The model under review builds one solid part; all positions refer to its coordinate system, in mm. A direction names the side the tool comes from. Round coordinates to 2 decimals unless told otherwise and drop trailing zeros. Write each loop counter-clockwise with the first axis right and the second up, starting at its lowest first coordinate (ties: lowest second). Pieces come first, ordered by that corner, then holes. Notation, with made-up numbers: (-8.75, 11.5) -> (13.25, 11.5) arc R13 cw to (13.25, 18.5) -> close; hole circle Ø5 at (65.25, 79.25). An arc over 180 degrees is marked (long way). Return JSON: item names as keys, results as strings. Group by question number.
1. Clearance check with flat-ended pins moving along their axes: P1, Ø1.3, axis at x = 1, z = 11, coming from the -Y side; P2, Ø1.1, axis at x = -4.5, y = -1.5, coming from the -Z side; P3, Ø2, axis at x = -3, z = 10, coming from the +Y side. State where each tip first meets the part, or that it passes through.
2. Tool access review of faces 5 (the flat face through (4, -1, 12)), 6 (the flat face through (4.5, -1, 11)), 7 (the flat face through (-5, 0, 12)): name each direction out of +Z, -Z, +X, -X, +Y, -Y from which nothing blocks a thin tool from reaching the whole face with its end or side.
3. Take a section at B-B, the plane z = 10.75. Write out the cut boundary in (x, y), then the cut area to 3 significant figures.
4. Mouldability with a two-part tool opening along X and no side actions: class faces 1 (the cylindrical face through (0, 1, 11)), 2 (the flat face through (4.5, -2, 12.2)), 3 (the flat face through (5, 0, 12)), 4 (the flat face through (-4, -1, 12)) as pulls with the +X half, pulls with the -X half, needs draft (parallel to the pull), parting line crosses it, or undercut.
5. For line 1 along X through (y, z) = (-1.8, 12.65); line 2 along Y through (x, z) = (-3, 13.5); line 3 along Z through (x, y) = (0.25, 0.8), list the stretches that pass through material, from the lowest coordinate up. Write a range as from..to.
6. Take a section at C-C, the plane z = 11.75. Write out the cut boundary in (x, y), then the cut area to 3 significant figures.
7. Take a section at A-A, the plane y = -1.45. Write out the cut boundary in (x, z), then the cut area to 3 significant figures.
8. Take a section at D-D, the plane x = 3. Write out the cut boundary in (y, z).
from build123d import *

# Parameters (mm, degrees)
BOSS_EXTRUDE1_DEPTH = 2
BOSS_EXTRUDE2_DEPTH = 2


with BuildPart() as part:
    # Sketch1 → Boss-Extrude1 (new body)
    with BuildSketch(Plane(origin=(0, 0, 0), x_dir=(1, 0, 0), z_dir=(0, 1, 0))):
        with BuildLine():
            Line((-5, -9.797958971), (-5, -13.076696831))
            ThreePointArc((-5, -13.076696831), (0, -14), (5, -13.076696831))
            Line((5, -13.076696831), (5, -9.797958971))
            ThreePointArc((5, -9.797958971), (0, -11), (-5, -9.797958971))
        make_face()
    extrude(amount=BOSS_EXTRUDE1_DEPTH)

    # Sketch3 → Boss-Extrude2 (add)
    with BuildSketch(Plane.XZ):
        with BuildLine():
            Line((5, 13.076696831), (5, 11))
            Line((5, 11), (4, 11))
            Line((4, 11), (4, 13.416407865))
            ThreePointArc((4, 13.416407865), (4.503204514, 13.255985407), (5, 13.076696831))
        make_face()
        with BuildLine():
            Line((-5, 11), (-5, 13.076696831))
            ThreePointArc((-5, 13.076696831), (-4.503204514, 13.255985407), (-4, 13.416407865))
            Line((-4, 13.416407865), (-4, 11))
            Line((-4, 11), (-5, 11))
        make_face()
    extrude(amount=BOSS_EXTRUDE2_DEPTH)


solid = part.part
Output:
{
 "1": {"P1": "stops at y = 0", "P2": "stops at z = 11", "P3": "stops at y = 2"},
 "2": {"face 5": "+Z, -Z, -Y", "face 6": "-Z, +X, -X, -Y", "face 7": "+Z, -Z, -X, +Y, -Y"},
 "3": {"outline": "(-5, 0) -> (-2.33, 0) -> (-2.33, 2) -> (-5, 2) -> close; (2.33, 0) -> (5, 0) -> (5, 2) -> (2.33, 2) -> close", "area": "10.7 mm^2"},
 "4": {"face 1": "undercut", "face 2": "needs draft", "face 3": "pulls with the +X half", "face 4": "undercut"},
 "5": {"line 1": "x = -5..-4, 4..5", "line 2": "y = 0..2", "line 3": "z = 11..14"},
 "6": {"outline": "(-5, -2) -> (-4, -2) -> (-4, 0) -> (4, 0) -> (4, -2) -> (5, -2) -> (5, 2) -> (-5, 2) -> close", "area": "24.0 mm^2"},
 "7": {"outline": "(-5, 11) -> (-4, 11) -> (-4, 13.42) arc R14 ccw to (-5, 13.08) -> close; (4, 11) -> (5, 11) -> (5, 13.08) arc R14 ccw to (4, 13.42) -> close", "area": "4.51 mm^2"},
 "8": {"outline": "(0, 10.58) -> (2, 10.58) -> (2, 13.67) -> (0, 13.67) -> close"}
}
